```python
from build123d import *

# Parameters (mm, degrees)
BOSS_EXTRUDE1_DEPTH = 5
CUT_EXTRUDE1_DEPTH  = 5
SKETCH5_R           = 4
SKETCH5_R_2         = 2
BOSS_EXTRUDE2_DEPTH = 5
SKETCH6_R           = 2
CUT_EXTRUDE2_DEPTH  = 5


with BuildPart() as part:
    # Sketch1 → Boss-Extrude1 (new body)
    with BuildSketch(Plane.XY):
        Polygon((7.5, 32.5), (7.5, 37.5), (-7.5, 37.5), (-7.5, 32.5), (-30, 32.5), (-30, -32.5), (30, -32.5), (30, 32.5), align=None)
    extrude(amount=BOSS_EXTRUDE1_DEPTH)

    # Sketch3 → Cut-Extrude1 (cut)
    with BuildSketch(Plane.XY.offset(5)):
        Polygon((30, 24.5), (25, 24.5), (25, 26), (21.6, 26), (21.6, 24.5), (10, 24.5), (10, 20.1), (21.6, 20.1), (21.6, 18.6), (25, 18.6), (25, 20.1), (30, 20.1), align=None)
        Polygon((30, -24.5), (30, -20.1), (25, -20.1), (25, -18.6), (21.6, -18.6), (21.6, -20.1), (10, -20.1), (10, -24.5), (21.6, -24.5), (21.6, -26), (25, -26), (25, -24.5), align=None)
        Polygon((-30, -24.5), (-25, -24.5), (-25, -26), (-21.6, -26), (-21.6, -24.5), (-10, -24.5), (-10, -20.1), (-21.6, -20.1), (-21.6, -18.6), (-25, -18.6), (-25, -20.1), (-30, -20.1), align=None)
    extrude(amount=-CUT_EXTRUDE1_DEPTH, mode=Mode.SUBTRACT)

    # Sketch5 → Boss-Extrude2 (add)
    with BuildSketch(Plane.XY.offset(5)):
        with Locations((0, -32.5)):
            Circle(SKETCH5_R)
        with Locations((0, -32.5)):
            Circle(SKETCH5_R_2, mode=Mode.SUBTRACT)
    extrude(amount=-BOSS_EXTRUDE2_DEPTH)

    # Sketch6 → Cut-Extrude2 (cut)
    with BuildSketch(Plane.XY.offset(5)):
        with Locations((0, -32.5)):
            Circle(SKETCH6_R)
    extrude(amount=-CUT_EXTRUDE2_DEPTH, mode=Mode.SUBTRACT)


solid = part.part
```
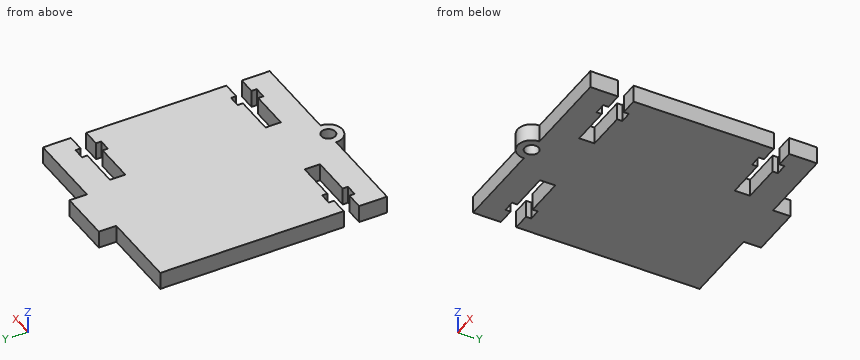
Geometry: final body of the model. Coordinates: model frame, mm. Coordinates: 2 decimals unless noted, no trailing zeros. Write each loop counter-clockwise with the first axis right and the second up, starting at its lowest first coordinate (ties: lowest second). Pieces come first, ordered by that corner, then holes. Notation, with made-up numbers: M -27,62.25 L 20,62.25 A20 cw 20,70.25 Z; hole C -28,17.5 d11. An arc over 180 degrees is marked long. Use CSV: the item, a comma, the result in double quotes. Start each with the question number.
1. Cut plane C-C on x = -14. Return the cut outline in (y, z).
2. Cut plane B-B on x = 0. Return the cut outline in (y, z).
3. Ray query, probe 1 along Y at (x, z) = (19, 4.75); probe 2 along X at (y, z) = (-25, 0.65); probe 3 along Y at (x, z) = (22.5, 0.45). Return the intervals inside material, ascending.
4. Cut plane A-A on x = 26. Return the cut outline in (y, z).
5. First-contact query: P1, Ø3, axis at x = 16, z = 3.5, coming from the +Y side; P2, Ø1.5, axis at x = 19.5, z = 2, coming from the -Y side; P3, Ø1.3, axis at y = 22, z = 1.5, coming from the +X side. Flat tips, straight axial feed; report the tip coordinate or a pass-through.
Entries:
1,outline,"M -32.5,0 L -24.5,0 L -24.5,5 L -32.5,5 Z; M -20.1,0 L 32.5,0 L 32.5,5 L -20.1,5 Z"
2,outline,"M -36.5,0 L -34.5,0 L -34.5,5 L -36.5,5 Z; M -30.5,0 L 37.5,0 L 37.5,5 L -30.5,5 Z"
3,probe 1,"-32.5 to -24.5, -20.1 to 20.1, 24.5 to 32.5"
3,probe 2,"-30 to -25, -21.6 to 21.6, 25 to 30"
3,probe 3,"-32.5 to -26, -18.6 to 18.6, 26 to 32.5"
4,outline,"M -32.5,0 L -24.5,0 L -24.5,5 L -32.5,5 Z; M -20.1,0 L 20.1,0 L 20.1,5 L -20.1,5 Z; M 24.5,0 L 32.5,0 L 32.5,5 L 24.5,5 Z"
5,P1,"y = 32.5"
5,P2,"y = -32.5"
5,P3,"x = 10"
